For this review, take the finished solid that the model builds, in its own axes (mm). A direction names the side the tool comes from. Coordinates: 2 decimals unless noted, no trailing zeros. Write each loop counter-clockwise with the first axis right and the second up, starting at its lowest first coordinate (ties: lowest second). Pieces come first, ordered by that corner, then holes.
1) Mouldability with a two-part tool opening along Y and no side actions: class faces 4 (the face through (-14.274, 0.628, 6.261)), 5 (the face through (-257, 119.275, 6)), 6 (the face through (-203.2, 167, 6)), 7 (the face through (-293.66, 59.92, 6.26)) as pulls with the +Y half, pulls with the -Y half, needs draft (parallel to the pull), parting line crosses it, or undercut.
2) Insertion check: P1, Ø3, axis at y = 159, z = 8, coming from the -X side; P2, Ø1.9, axis at y = 58, z = 8, coming from the +X side; P3, Ø7, axis at y = 201, z = 4.5, coming from the +X side. Each pin has a flat end and moves straight along its axis. Give the tip position at first contact, or say it passes through.
3) We need section D-D on x = 93. Write out the cut boundary in (y, z), then the cut area to 3 significant figures.
4) To check wall thickness, follow line 1 along Y through (x, z) = (154, 11.5); line 2 along X through (y, z) = (72.5, 8.5); line 3 along Y through (x, z) = (57, 7.5). State the ranges of each line that lie inside material, in increasing order.
5) We need section A-A on x = -260.35. Write out the cut boundary in (y, z).
6) For faces 1 (the face through (-307.331, 115.654, 6.439)), 2 (the face through (166, -40, 6.35)), 3 (the face through (-255, -20.425, 6)), list the 3-axis set-ups (+Z, -Z, +X, -X, +Y, -Y) from which the entire face can be reached by the end or side of a thin tool; tool diameter is ignored.
7) We need section C-C on y = -164. Write out the cut boundary in (x, z).
8) We need section B-B on z = 10.75. Give the number of separate pieces and of enclosed holes in the cut face, then the cut area to 3 significant figures.
from build123d import *

# Parameters (mm, degrees)
SKETCH1_W               = 406.4
SKETCH1_H               = 406.4
SKETCH1_R               = 14.2875
BOSS_EXTRUDE1_DEPTH     = 12.7
CUT_EXTRUDE1_DEPTH      = 6.35
CUT_EXTRUDE2_DEPTH      = 13.7
SKETCH4_R               = 3.175
CUT_EXTRUDE3_DEPTH      = 1
CUT_EXTRUDE3_DEPTH_BACK = 13.7
SKETCH6_W               = 108.979085312
SKETCH6_H               = 139.7
SKETCH6_R               = 34.925
SKETCH6_R_2             = 3.175
BOSS_EXTRUDE2_DEPTH     = 12.7
FILLET1_R               = 12.7


with BuildPart() as part:
    # Sketch1 → Boss-Extrude1 (new body)
    with BuildSketch(Plane.XY):
        Rectangle(SKETCH1_W, SKETCH1_H)
        Circle(SKETCH1_R, mode=Mode.SUBTRACT)
    extrude(amount=BOSS_EXTRUDE1_DEPTH)

    # Sketch2 → Cut-Extrude1 (cut)
    with BuildSketch(Plane.XY.offset(12.7)):
        with BuildLine():
            Line((-18.027683557, 172.095842576), (-17.696900373, 168.938120694))
            ThreePointArc((-17.696900373, 168.938120694), (126.212734393, -113.68207679), (-169.8625, 0))
            Line((-169.8625, 0), (-169.8625, 203.2))
            Line((-169.8625, 203.2), (-173.0375, 203.2))
            Line((-173.0375, 203.2), (-173.0375, 0))
            ThreePointArc((-173.0375, 0), (128.571850923, -115.806975422), (-18.027683557, 172.095842576))
        make_face()
    extrude(amount=-CUT_EXTRUDE1_DEPTH, mode=Mode.SUBTRACT)

    # Sketch3 → Cut-Extrude2 (cut, through all)
    with BuildSketch(Plane.XY.offset(12.7)):
        with BuildLine():
            Line((58.432704894, 203.2), (58.432704894, 194.617211466))
            ThreePointArc((58.432704894, 194.617211466), (163.039513149, 121.278015948), (203.2, -3.13e-07))
            Line((203.2, -3.13e-07), (203.2, 203.2))
            Line((203.2, 203.2), (58.432704894, 203.2))
        make_face()
        with BuildLine():
            Line((203.2, -203.2), (203.2, -3.13e-07))
            ThreePointArc((203.2, -3.13e-07), (143.684097934, -143.68409794), (3.04e-07, -203.2))
            Line((3.04e-07, -203.2), (203.2, -203.2))
        make_face()
        with BuildLine():
            Line((-203.2, -203.2), (3.04e-07, -203.2))
            ThreePointArc((3.04e-07, -203.2), (-143.68409783, -143.684098045), (-203.2, 0))
            Line((-203.2, 0), (-203.2, -203.2))
        make_face()
    extrude(amount=-CUT_EXTRUDE2_DEPTH, mode=Mode.SUBTRACT)

    # Sketch4 → Cut-Extrude3 (cut, two sides)
    with BuildSketch(Plane.XY.offset(12.7)) as cut_extrude3_sk:
        with Locations((-190.5, 190.5)):
            Circle(SKETCH4_R)
        with Locations((-164.977839421, -95.25)):
            Circle(SKETCH4_R)
        with Locations((164.977839421, -95.25)):
            Circle(SKETCH4_R)
        with Locations((0, 190.5)):
            Circle(SKETCH4_R)
    extrude(amount=CUT_EXTRUDE3_DEPTH, mode=Mode.SUBTRACT)
    extrude(cut_extrude3_sk.sketch, amount=-CUT_EXTRUDE3_DEPTH_BACK, mode=Mode.SUBTRACT)

    # Sketch6 → Boss-Extrude2 (add, through all)
    with BuildSketch(Plane(origin=(0, 0, 0), x_dir=(-1, 0, 0), z_dir=(0, 0, -1))):
        with Locations((256.660457344, 49.425474201)):
            Rectangle(SKETCH6_W, SKETCH6_H)
        with Locations((260.35, 49.425474201)):
            Circle(SKETCH6_R, mode=Mode.SUBTRACT)
        with Locations((234.95, 106.575474201)):
            Circle(SKETCH6_R_2, mode=Mode.SUBTRACT)
        with Locations((285.75, 106.575474201)):
            Circle(SKETCH6_R_2, mode=Mode.SUBTRACT)
        with Locations((285.75, -7.724525799)):
            Circle(SKETCH6_R_2, mode=Mode.SUBTRACT)
        with Locations((234.95, -7.724525799)):
            Circle(SKETCH6_R_2, mode=Mode.SUBTRACT)
    extrude(amount=-BOSS_EXTRUDE2_DEPTH)

    # Fillet1
    fillet1_edges = [part.edges().sort_by_distance(p)[0] for p in [
        (-202.170914688, -20.424525799, 6.35),
        (-311.15, 119.275474201, 6.35),
        (-311.15, -20.424525799, 6.35),
        (-203.2, 119.275474201, 6.35),
    ]]
    fillet(fillet1_edges, radius=FILLET1_R)


solid = part.part
Result:
1. face 4: undercut
1. face 5: pulls with the +Y half
1. face 6: needs draft
1. face 7: undercut
2. P1: stops at x = -203.2
2. P2: stops at x = 195.03
2. P3: stops at x = 58.43
3. outline: (-180.67, 0) - (180.67, 0) - (180.67, 12.7) - (145.92, 12.7) - (145.92, 6.35) - (142.14, 6.35) - (142.14, 12.7) - (-142.14, 12.7) - (-142.14, 6.35) - (-145.92, 6.35) - (-145.92, 12.7) - (-180.67, 12.7) - close
3. area: 4,540 mm2
4. line 1: y = -132.57 to -78.9, -71.67 to 71.67, 78.9 to 132.57
4. line 2: x = -311.15 to -286.57, -234.13 to -173.04, -169.86 to 153.61, 157.12 to 189.83
4. line 3: y = -195.04 to -163.38, -160.01 to 160.01, 163.38 to 203.2
5. outline: (-20.42, 0) - (14.5, 0) - (14.5, 12.7) - (-20.42, 12.7) - close; (84.35, 0) - (119.28, 0) - (119.28, 12.7) - (84.35, 12.7) - close
6. face 1: +Z, -Z, -X, +Y
6. face 2: +Z
6. face 3: +Z, -Z, -X, -Y
7. outline: (-119.98, 0) - (119.98, 0) - (119.98, 12.7) - (55.19, 12.7) - (55.19, 6.35) - (44.24, 6.35) - (44.24, 12.7) - (-44.24, 12.7) - (-44.24, 6.35) - (-55.19, 6.35) - (-55.19, 12.7) - (-119.98, 12.7) - close
8. separate pieces: 1
8. enclosed holes: 10
8. area: 146,000 mm2
